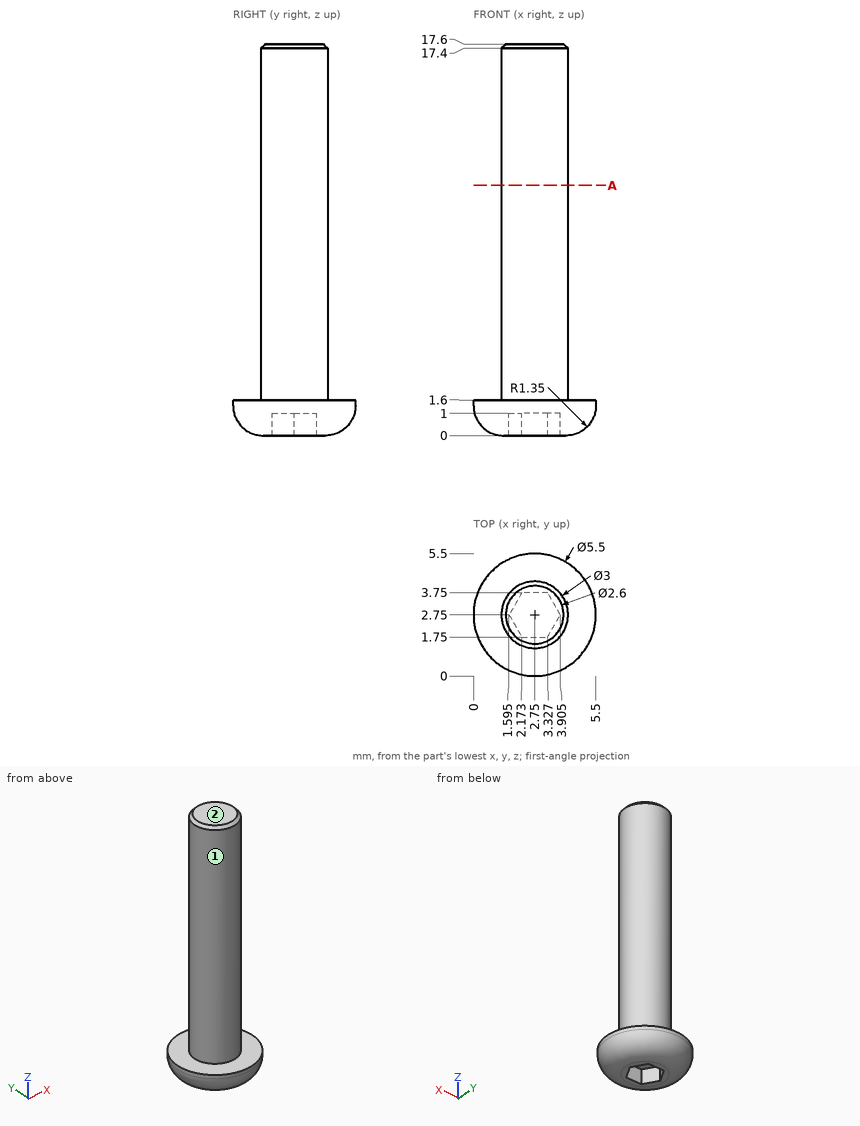
Geometry: see drawing. Coordinates: mm, zero at the bounding-box minimum. Round coordinates to 2 decimals unless told otherwise and drop trailing zeros. Loops run counter-clockwise (first coordinate to the right, second up) from the corner with the lowest first, then second, coordinate; pieces in that order, holes last. Notation, with made-up numbers: (13, 26) - (44, 26) arc R16 cw to (44, 39) - close; hole circle Ø4 at (70.25, 82). An arc over 180 degrees is marked (long way). One line per item, written item: value. Start each with the question number.
(1) Draft query along X for the marked faces 1 and 2. Return one class per face: +X half, -X half, draft (parallel to the pull), parting line (faces both ways), or undercut.
(2) Contact query for flat-ended pins moving along their axis: P1, Ø1, axis at x = 3, y = 5, coming from the +Z side; P2, Ø3, axis at x = 3.5, y = 4, coming from the +Z side; P3, Ø2, axis at x = 5, y = 5, coming from the -Z side; P4, Ø3, axis at x = 4, z = 11, coming from the +Y side. Output: stop coordinate, or through.
(3) Section A-A, the plane z = 11.25. Return loops of the section in (x, y).
(4) Ray query, line 1 (Y direction, x = 3.3, z = 6.75) (1 decimal); line 2 (Y direction, x = 2.65, z = 5). Return the intervals inside material, ascending. Write a range as [from, to].
Results below:
1. face 1: parting line
1. face 2: draft
2. P1: z = 1.6
2. P2: z = 17.6
2. P3: z = 0.25
2. P4: y = 4.25
3. outline: circle Ø3 at (2.75, 2.75)
4. line 1: [1.4, 4.1]
4. line 2: [1.25, 4.25]
